from build123d import *

# Parameters (mm, degrees)
SCHIZZO1_R                   = 2.5
SCHIZZO1_R_2                 = 1.5
ESTRUSIONE_ESTRUSIONE1_DEPTH = 5
SCHIZZO2_R                   = 2.75
ESTRUSIONE_ESTRUSIONE2_DEPTH = 2
RACCORDO1_R                  = 1


with BuildPart() as part:
    # Schizzo1 → Estrusione-Estrusione1 (new body)
    with BuildSketch(Plane.XY):
        Circle(SCHIZZO1_R)
        Circle(SCHIZZO1_R_2, mode=Mode.SUBTRACT)
    extrude(amount=ESTRUSIONE_ESTRUSIONE1_DEPTH)

    # Schizzo2 → Estrusione-Estrusione2 (add)
    with BuildSketch(Plane.XY.offset(5)):
        Circle(SCHIZZO2_R)
    extrude(amount=ESTRUSIONE_ESTRUSIONE2_DEPTH)

    # Raccordo1
    # the kernel refuses this fillet: 1 mm, written as the material it adds along each edge
    with BuildSketch(Plane(origin=(0, 0, 5), x_dir=(1, 0, 0), z_dir=(0, -1, 0))) as raccordo1_piece_1:
        with BuildLine():
            CenterArc((3.5, -0.661437828), RACCORDO1_R, 138.590377891, 41.409622109)
            Line((2.5, -0.661437828), (2.48, -0.661437828))
            Line((2.48, -0.661437828), (2.48, 0))
            Line((2.48, 0), (2.5, 0.02))
            ThreePointArc((2.5, 0.02), (2.625, 0.02), (2.735, 0.013228757))
            Line((2.735, 0.013228757), (2.75, 0))
        make_face()
    revolve(axis=Axis((0, 0, 5), (0, 0, 1)))


solid = part.part
Geometry check sheet. Reference: the model listing, model coordinates, mm. Give positions to 0.01 mm unless a question says otherwise; leave off trailing zeros. Loops run counter-clockwise (first coordinate to the right, second up) from the corner with the lowest first, then second, coordinate; pieces in that order, holes last. Notation, with made-up numbers: M 5,64.25 L 33,64.25 A24 cw 33,103.25 Z; hole C 53,36 d8. An arc over 180 degrees is marked long. Answer as a JSON object with one key per item and string values. Group by question number.
Item 1: Sectioned sample at D-D on z = 5.5. Record the boundary of the cut face in (x, y).
Item 2: Mould release check, pull along X, two halves, no side actions. Record for faces 1 (the flat face through (0, 0, 5)), 2 (the cylindrical face through (-1.5, 0.07, 2.46)), 3 (the cylindrical face through (-0.54, -2.44, 2.14)), 4 (the flat face through (0, -2, 0)): pulls with the +X half, pulls with the -X half, needs draft (parallel to the pull), parting line crosses it, or undercut.
Item 3: Gauge pin test, flat ends, axial feed: pin 1 (1.5 mm diameter, centred on y = 2, z = 2, fed in from +X); pin 2 (0.9 mm diameter, centred on x = 0, y = -0.5, fed in from -Z). Record the tip position at first contact, or that the pin passes through.
Item 4: Material ranges on L1, parallel to Y at x = 0, z = 1.5; L2, parallel to X at y = 1.35, z = 4.5; L3, parallel to X at y = -0.4, z = 4.5, recorded low to high.
Item 5: Sectioned sample at C-C on z = 1. Record the boundary of the cut face in (x, y), plus the area to 3 significant figures.
Item 6: Sectioned sample at A-A on x = 0. Record the boundary of the cut face in (y, z), plus the area to 3 significant figures.
Findings below:
{
 "1": {"outline": "C 0,0 d5.5"},
 "2": {"face 1": "undercut", "face 2": "undercut", "face 3": "parting line crosses it", "face 4": "needs draft"},
 "3": {"pin 1": "x = 2.17", "pin 2": "z = 5"},
 "4": {"L1": "-2.5 to -1.5, 1.5 to 2.5", "L2": "-2.12 to -0.65, 0.65 to 2.12", "L3": "-2.48 to -1.45, 1.45 to 2.48"},
 "5": {"outline": "C 0,0 d5; hole C 0,0 d3", "area": "12.6 mm2"},
 "6": {"outline": "M -2.75,5 A1 cw -2.5,4.34 L -2.5,0 L -1.5,0 L -1.5,5 L 1.5,5 L 1.5,0 L 2.5,0 L 2.5,4.34 A1 cw 2.75,5 L 2.75,7 L -2.75,7 Z", "area": "21.1 mm2"}
}
